from build123d import *

# Parameters (mm, degrees)
BOSS_EXTRUDE1_DEPTH             = 2.175
F_2_CLEARANCE_HOLE2_D           = 2.2606
F_2_CLEARANCE_HOLE2_CSINK_D     = 3.7084
F_2_CLEARANCE_HOLE2_CSINK_ANGLE = 90


with BuildPart() as part:
    # Sketch1 → Boss-Extrude1 (new, symmetric)
    with BuildSketch(Plane(origin=(0, 0, 0), x_dir=(0, 0, -1), z_dir=(1, 0, 0))):
        with BuildLine():
            Line((-10.101597565, 8.379005111), (-11.5955, 4.668445111))
            ThreePointArc((-11.5955, 4.668445111), (0, -12.5), (11.5955, 4.668445111))
            Line((11.5955, 4.668445111), (10.101597565, 8.379005111))
            ThreePointArc((10.101597565, 8.379005111), (9.860779562, 6.11162847), (8.0955, 4.668445111))
            Line((8.0955, 4.668445111), (-8.0955, 4.668445111))
            ThreePointArc((-8.0955, 4.668445111), (-9.860779562, 6.11162847), (-10.101597565, 8.379005111))
        make_face()
    extrude(amount=BOSS_EXTRUDE1_DEPTH, both=True)

    # #2 Clearance Hole2 (through all)
    with Locations(Plane(origin=(2.175, 0.668445111, 3.535533906), x_dir=(0, 0, 1), z_dir=(1, 0, 0))):
        with Locations((0, 0), (-7.071067812, 7.071067812)):
            CounterSinkHole(F_2_CLEARANCE_HOLE2_D / 2, F_2_CLEARANCE_HOLE2_CSINK_D / 2, counter_sink_angle=F_2_CLEARANCE_HOLE2_CSINK_ANGLE)


solid = part.part
The listing builds one solid part. Answer for the finished solid, in the listing's coordinates (mm). A direction names the side the tool comes from. Coordinates: 2 decimals unless noted, no trailing zeros. Loops run counter-clockwise (first coordinate to the right, second up) from the corner with the lowest first, then second, coordinate; pieces in that order, holes last. Notation, with made-up numbers: (31.25, 70) -> (78.25, 70) arc R18 ccw to (78.25, 75) -> close; hole circle Ø6 at (60.5, -38). An arc over 180 degrees is marked (long way). Write item = value, one per line. Start each with the question number.
1) Given pin 1 Ø2 at (x, z) = (-1, 3) entering from +Y; pin 2 Ø3.5 at (y, z) = (-6.4, -3.54) entering from -X (3 decimals); pin 3 Ø1 at (x, z) = (-1.5, 3.5) entering from -Y; pin 4 Ø1.5 at (x, y) = (0, 4) entering from -Z, each flat-ended and moving along its own axis, determine where each tip first touches the part or whether it passes through.
2) A cutting plane is placed at B-B (x = -0.6). Give the vertices of the cut face in (y, z), then the cut area to 3 significant figures.
3) A cutting plane is placed at A-A (y = 6.5). Give the vertices of the cut face in (x, z) (3 decimals), then the cut area to 3 significant figures.
4) A cutting plane is placed at C-C (z = 0). Give the vertices of the cut face in (x, y) (3 decimals), then the cut area to 3 significant figures.
5) A cutting plane is placed at D-D (y = -9.25). Give the vertices of the cut face in (x, z) (3 decimals).
6) Straight lines are drawn through the part: line 1 (Z direction, x = -1.15, y = 7); line 2 (Y direction, x = 0.35, z = 3.5); line 3 (Z direction, x = 0.7, y = 1.25). For each, find the intervals that lie inside material, in ascending order. Write a range as from..to.
7) A tool of negligible diameter and unlimited length cuts with its end or side. For faces 4 (the face through (0.03, 6.141, -9.876)), 5 (the face through (0, 4.668, 0)), 6 (the face through (2.175, -2, 0)), from which of +Z, -Z, +X, -X, +Y, -Y can it reach the whole face along a straight path? Write none if from no direction.
8) The mould has two halves that part along Y. Classify faces 1 (the face through (-2.175, -2, 0)), 2 (the face through (0.03, 6.5, -10.86)), 3 (the face through (0.03, 6.083, 9.845)): released by +Y, released by -Y, zero draft, split by the parting line, or undercut.
Responses:
q1.pin_1 = 4.67
q1.pin_2 = -2.175
q1.pin_3 = -12.13
q1.pin_4 = -12.07
q2.outline = (4.67, -11.6) -> (8.38, -10.1) arc R3 cw to (4.67, -8.1) -> (4.67, 8.1) arc R3 cw to (8.38, 10.1) -> (4.67, 11.6) arc R12.5 ccw (long way) to start; hole circle Ø2.26 at (-6.4, -3.54); hole circle Ø2.26 at (0.67, 3.54)
q2.area = 359 mm²
q3.outline = (-2.175, -10.858) -> (2.175, -10.858) -> (2.175, -10.036) -> (-2.175, -10.036) -> close; (-2.175, 10.036) -> (2.175, 10.036) -> (2.175, 10.858) -> (-2.175, 10.858) -> close
q3.area = 7.15 mm²
q4.outline = (-2.175, -12.5) -> (2.175, -12.5) -> (2.175, 4.668) -> (-2.175, 4.668) -> close
q4.area = 74.7 mm²
q5.outline = (-2.175, -8.408) -> (2.175, -8.408) -> (2.175, 8.408) -> (-2.175, 8.408) -> close
q6.line_1 = -10.66..-10.17, 10.17..10.66
q6.line_2 = -12..-0.46, 1.8..4.67
q6.line_3 = -12.44..2.57, 4.5..12.44
q7.face_4 = +X, -X
q7.face_5 = +X, -X, +Y
q7.face_6 = +Z, -Z, +X, +Y, -Y
q8.face_1 = zero draft
q8.face_2 = released by +Y
q8.face_3 = undercut
